For this review, use the dimensioned drawing (mm, ordinates from the lowest corner) and the shaded views. A direction names the side the tool comes from. Coordinates: 2 decimals unless noted, no trailing zeros. Write each loop counter-clockwise with the first axis right and the second up, starting at its lowest first coordinate (ties: lowest second). Pieces come first, ordered by that corner, then holes.
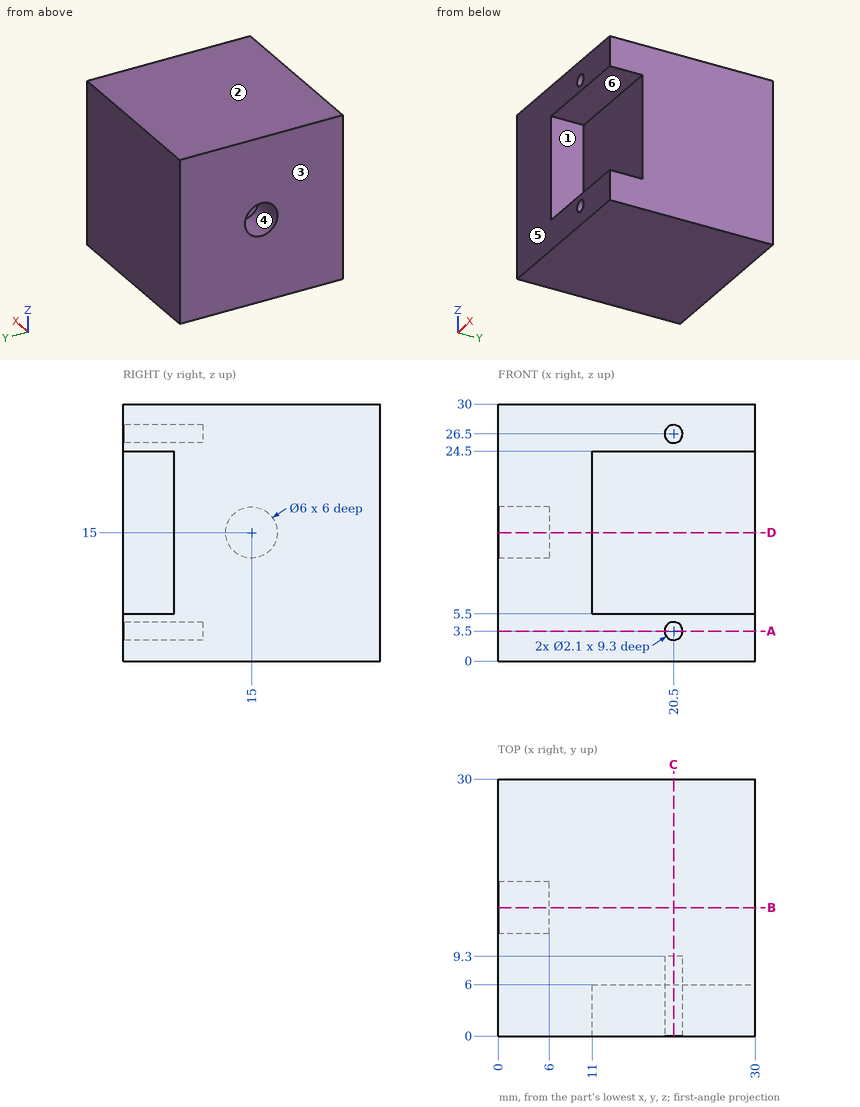
Item 1: Machinability: for the marked faces 4, 5 and 6, which of the approach directions +Z, -Z, +X, -X, +Y, -Y give a long, thin tool a straight path to every point of the face, cutting with its end or side? Answer none if there is none.
Solved:
face 4: -X
face 5: +Z, -Z, +X, -X, -Y
face 6: +X, -Y
Item 2: Take a section at B-B, the plane y = 15. Write out the cut boundary in (x, z), plus the area to 3 significant figures.
Solved:
outline: (0, 0) - (30, 0) - (30, 30) - (0, 30) - (0, 18) - (6, 18) - (6, 12) - (0, 12) - close
area: 864 mm2
Item 3: Mouldability with a two-part tool opening along Z and no side actions: class the marked faces 1, 2 and 3 as pulls with the +Z half, pulls with the -Z half, needs draft (parallel to the pull), parting line crosses it, or undercut.
Solved:
face 1: undercut
face 2: pulls with the +Z half
face 3: needs draft
Item 4: For pin 1 (2.5 mm diameter, centred on x = 21, z = 4, fed in from -Y), flat-tipped, find the tip position at first contact; note if it passes through.
Solved:
pin 1: stops at y = 0
Item 5: Take a section at A-A, the plane z = 3.5. Write out the cut boundary in (x, y), plus the area to 3 significant figures.
Solved:
outline: (0, 0) - (19.45, 0) - (19.45, 9.3) - (21.55, 9.3) - (21.55, 0) - (30, 0) - (30, 30) - (0, 30) - close
area: 880 mm2
Item 6: To check wall thickness, follow line 1 along Z through (x, y) = (20.5, 4.5); line 2 along Z through (x, y) = (4.7, 15); line 3 along Y through (x, z) = (23.25, 11). State the ranges of each line that lie inside material, in increasing order.
Solved:
line 1: z = 0 to 2.45, 4.55 to 5.5, 24.5 to 25.45, 27.55 to 30
line 2: z = 0 to 12, 18 to 30
line 3: y = 6 to 30
Item 7: Take a section at C-C, the plane x = 20.5. Write out the cut boundary in (y, z), plus the area to 3 significant figures.
Solved:
outline: (0, 0) - (30, 0) - (30, 30) - (0, 30) - (0, 27.55) - (9.3, 27.55) - (9.3, 25.45) - (0, 25.45) - (0, 24.5) - (6, 24.5) - (6, 5.5) - (0, 5.5) - (0, 4.55) - (9.3, 4.55) - (9.3, 2.45) - (0, 2.45) - close
area: 747 mm2
Item 8: Take a section at D-D, the plane z = 15. Write out the cut boundary in (x, y).
Solved:
outline: (0, 0) - (11, 0) - (11, 6) - (30, 6) - (30, 30) - (0, 30) - (0, 18) - (6, 18) - (6, 12) - (0, 12) - close
